```python
from build123d import *

# Parameters (mm, degrees)
SKETCH1_R           = 2.75
BOSS_EXTRUDE1_DEPTH = 6
BODY_START          = -3
SKETCH2_R           = 2.75
BODY_HOLE_DEPTH     = 3
POT_START           = -3
POT_INSERT_DEPTH    = 2.5
CUT_EXTRUDE2_DEPTH  = 23.226110771
CUT_REVOLVE1_ANGLE  = 180
SKETCH7_R           = 0.8
SCREW_HOLES_DEPTH   = 22.656407828
SKETCH9_R           = 1.25
SCREW_HEADS_DEPTH   = 4


with BuildPart() as part:
    # Sketch1 → Boss-Extrude1 (new body)
    with BuildSketch(Plane.XY):
        with BuildLine():
            Line((17, -12), (17, 12))
            Line((17, 12), (5, 12))
            ThreePointArc((5, 12), (-13, 0), (5, -12))
            Line((5, -12), (17, -12))
        make_face()
        Circle(SKETCH1_R, mode=Mode.SUBTRACT)
    extrude(amount=-BOSS_EXTRUDE1_DEPTH)

    # Sketch2 → Body Hole (cut)
    with BuildSketch(Plane.XY.offset(BODY_START)):
        with BuildLine():
            ThreePointArc((5, 12), (-13, 0), (5, -12))
            Line((5, -12), (13, -12))
            Line((13, -12), (13, -4.25))
            Line((13, -4.25), (17, -4.25))
            Line((17, -4.25), (17, 4.25))
            Line((17, 4.25), (13, 4.25))
            Line((13, 4.25), (13, 12))
            Line((13, 12), (5, 12))
        make_face()
        Circle(SKETCH2_R, mode=Mode.SUBTRACT)
    extrude(amount=-BODY_HOLE_DEPTH, mode=Mode.SUBTRACT)

    # Sketch8 → Pot Insert (cut)
    with BuildSketch(Plane(origin=(28.28760271, 0, 0), x_dir=(1, 0, 0), z_dir=(0, 0, 1)).offset(POT_START)):
        Polygon((-35.287602709, 0), (-35.287602709, -1.5), (-33.787602709, -1.5), (-32.287602709, -4.5), (-32.287602709, -5.5), (-28.287602709, -5.5), (-24.037602709, -5.5), (-24.037602709, -4.5), (-18.787602709, -4.5), (-18.787602709, 0), (-18.787602709, 4.5), (-24.037602709, 4.5), (-24.037602709, 5.5), (-28.287602709, 5.5), (-32.287602709, 5.5), (-32.287602709, 4.5), (-33.787602709, 1.5), (-35.287602709, 1.5), align=None)
    extrude(amount=POT_INSERT_DEPTH, mode=Mode.SUBTRACT)

    # Sketch3 → Cut-Extrude2 (cut, through all)
    with BuildSketch(Plane(origin=(0, 0, 0), x_dir=(0, 0, -1), z_dir=(1, 0, 0))):
        with BuildLine():
            ThreePointArc((-2, 0), (2.393398282, 10.606601718), (13, 15))
            Line((13, 15), (-2, 15))
            Line((-2, 15), (-2, 0))
        make_face()
        with BuildLine():
            ThreePointArc((13, -15), (2.393398282, -10.606601718), (-2, 0))
            Line((-2, 0), (-2, -15))
            Line((-2, -15), (13, -15))
        make_face()
    extrude(amount=CUT_EXTRUDE2_DEPTH, mode=Mode.SUBTRACT)

    # Sketch6 → Cut-Revolve1 (revolve, cut)
    with BuildSketch(Plane(origin=(0, 0, 0), x_dir=(0, 0, -1), z_dir=(1, 0, 0))):
        with BuildLine():
            ThreePointArc((-1, 5.385164807), (4.508164866, 12.36481848), (13, 15))
            Line((13, 15), (-2, 15))
            Line((-2, 15), (-2, 5.385164807))
            Line((-2, 5.385164807), (-1, 5.385164807))
        make_face()
    revolve(axis=Axis((0, 0, 0), (0, 0, 1)), revolution_arc=CUT_REVOLVE1_ANGLE, mode=Mode.SUBTRACT)

    # Sketch7 → Screw Holes (cut, through all)
    with BuildSketch(Plane.XY):
        with Locations((15, 10)):
            Circle(SKETCH7_R)
        with Locations((15, -10)):
            Circle(SKETCH7_R)
    extrude(amount=-SCREW_HOLES_DEPTH, mode=Mode.SUBTRACT)

    # Sketch9 → Screw Heads (cut)
    with BuildSketch(Plane.XY):
        with Locations((15, -10)):
            Circle(SKETCH9_R)
    extrude(amount=-SCREW_HEADS_DEPTH, mode=Mode.SUBTRACT)


solid = part.part
```
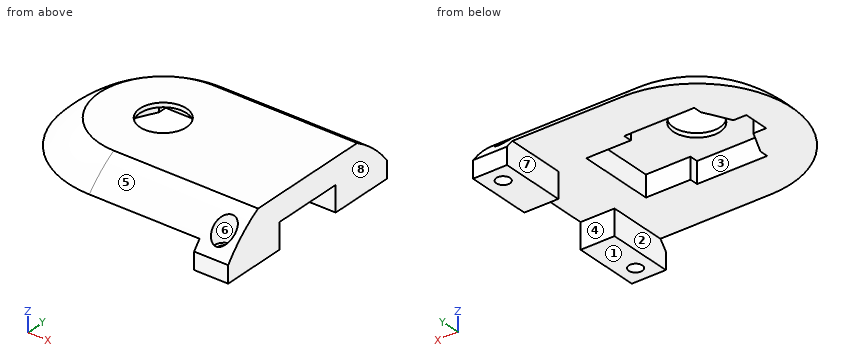
Geometry: final body of the model. Coordinates: model frame, mm. Face numbers are marked on the shaded views. A direction names the side the tool comes from. Give positions to 0.01 mm unless a question says otherwise; leave off trailing zeros. Loops run counter-clockwise (first coordinate to the right, second up) from the corner with the lowest first, then second, coordinate; pieces in that order, holes last. Notation, with made-up numbers: (51.5, -17) -> (107.5, -17) arc R21 ccw to (107.5, 13) -> close; hole circle Ø2 at (2, 71). An arc over 180 degrees is marked (long way). Use CSV: the item, a comma, the result in double quotes.
(1) First-contact query: P1, Ø0.8, axis at x = 1.5, z = -2, coming from the +Y side; P2, Ø1, axis at x = 15, y = 10, coming from the +Z side; P3, Ø1.5, axis at y = -9, z = -4.5, coming from the -X side; P4, Ø0.8, axis at y = -5, z = -1.5, coming from the -X side. Flat tips, straight axial feed; report the tip coordinate or a pass-through.
From the geometry:
P1,"y = 10.61"
P2,"through"
P3,"x = 13"
P4,"x = -8.81"
(2) Cut plane B-B (y = 0). Output: boundary loops of the cut face in (x, z), plus the area to 3 significant figures.
From the geometry:
outline,"(-11.18, -3) -> (-7, -3) -> (-7, -0.5) -> (-2.75, -0.5) -> (-2.75, 0) -> (-7.48, 0) arc R15 ccw to start; (2.75, -0.5) -> (9.5, -0.5) -> (9.5, -3) -> (17, -3) -> (17, 0) -> (2.75, 0) -> close"
area,"35.6 mm^2"
(3) Cut plane A-A (z = -5.25). Output: boundary loops of the cut face in (x, y).
From the geometry:
outline,"(13, -12) -> (17, -12) -> (17, -4.25) -> (13, -4.25) -> close; (13, 4.25) -> (17, 4.25) -> (17, 12) -> (13, 12) -> close; hole circle Ø1.6 at (15, -10); hole circle Ø1.6 at (15, 10)"
(4) Cut plane C-C (x = -0.5). Output: boundary loops of the cut face in (y, z).
From the geometry:
outline,"(-11.17, -3) -> (-5.5, -3) -> (-5.5, -0.5) -> (-2.7, -0.5) -> (-2.7, 0) -> (-7.47, 0) arc R14.99 ccw to start; (2.7, -0.5) -> (5.5, -0.5) -> (5.5, -3) -> (11.17, -3) arc R14.99 ccw to (7.47, 0) -> (2.7, 0) -> close"
(5) Pull-direction query (X, two-part tool) for the marked faces 6, 7 and 8; classes: released by +X, released by -X, zero draft, split by the parting line, or undercut.
From the geometry:
face 6,"undercut"
face 7,"released by -X"
face 8,"released by +X"
(6) Access query for the marked faces 1, 2, 3, 4 and 5. Directions: +Z, -Z, +X, -X, +Y, -Y. A direction counts if a zero-diameter tool reaches every point of the face in a straight line with its end or side. Return the directions, or none.
From the geometry:
face 1,"-Z, +X, -X, +Y, -Y"
face 2,"-Z, -X, +Y, -Y"
face 3,"-Z"
face 4,"-Z, +X, -X"
face 5,"+Z, +X, -X, -Y"
(7) Ray query, line 1 along Y through (x, z) = (15, -4.65); line 2 along X through (y, z) = (10, -4.45); line 3 along Y through (x, z) = (13.5, -4.75). Return the intervals inside material, ascending. Write a range as [from, to].
From the geometry:
line 1,"[-12, -10.8], [-9.2, -4.25], [4.25, 9.2], [10.8, 12]"
line 2,"[13, 14.2], [15.8, 17]"
line 3,"[-12, -4.25], [4.25, 12]"
(8) Cut plane D-D (x = 5.25). Output: boundary loops of the cut face in (y, z).
From the geometry:
outline,"(-11.18, -3) -> (-4.5, -3) -> (-4.5, -0.5) -> (4.5, -0.5) -> (4.5, -3) -> (11.18, -3) arc R15 ccw to (7.48, 0) -> (-7.48, 0) arc R15 ccw to start"
